```python
from build123d import *

# Parameters (mm, degrees)
F0_W      = 23.876
F0_H      = 22.352
F1_DEPTH  = 31.75
F2_R      = 0.796109
F3_DEPTH  = 25.4
F5_R      = 0.835635
F6_DEPTH  = 6.35
F7_R      = 0.804369
F4_W      = 23.876
F4_H      = 22.352
F4_R      = 0.796109
F8_DEPTH  = 6.35
F9_R      = 43.215518
F10_DEPTH = 127


with BuildPart() as f1:
    # F0 (on Top) → F1 (new body)
    with BuildSketch(Plane.XY):
        with Locations((11.938, -11.176)):
            Rectangle(F0_W, F0_H)
    extrude(amount=F1_DEPTH)

    # F2 (on face) → F3 (cut)
    with BuildSketch(Plane.XY.offset(31.75)):
        with Locations((22.537371, -1.488913)):
            Circle(F2_R)
    extrude(amount=-F3_DEPTH, mode=Mode.SUBTRACT)

    # F5 (on face) → F6 (cut)
    with BuildSketch(Plane.XY.offset(31.75)):
        with Locations((1.065723, -1.193718)):
            Circle(F5_R)
    extrude(amount=-F6_DEPTH, mode=Mode.SUBTRACT)

    # F7 (on face) + F4 (on face) → F8 (cut)
    with BuildSketch(Plane.XY.offset(31.75)):
        with Locations((1.000239, -21.275662)):
            Circle(F7_R)
    with BuildSketch(Plane.XY.offset(31.75)):
        with Locations((11.938, -11.176)):
            Rectangle(F4_W, F4_H)
        with Locations((22.537371, -1.488913)):
            Circle(F4_R, mode=Mode.SUBTRACT)
    extrude(amount=-F8_DEPTH, mode=Mode.SUBTRACT)

    # F9 (on Front) → F10 (join)
    with BuildSketch(Plane.XZ):
        with Locations((32.045215, 28.994571)):
            Circle(F9_R)
    extrude(amount=F10_DEPTH)


solid = f1.part
```
The listing builds one solid part. Answer for the finished solid, in the listing's coordinates (mm). Give positions to 0.01 mm unless a question says otherwise; leave off trailing zeros. Order: outer loops, then holes, each group sorted by start corner. A loop starts at its lowest first (then second) coordinate and runs counter-clockwise, first axis right, second up. Notation, with made-up numbers: (63, 54.5) -> (87, 54.5) arc R13 cw to (87, 65.5) -> close; hole circle Ø2 at (-2.5, -6.75). An arc over 180 degrees is marked (long way). Write each question's results on one line, items separated by ' | '.
Q1. Each of these flat-tipped pins is pushed along its axis until it touches: P1, Ø1.5, axis at x = 39.5, y = -105.5, coming from the -Z side; P2, Ø1.5, axis at x = 60, y = -90.5, coming from the +Z side; P3, Ø4, axis at x = 13, y = -60.5, coming from the -Z side. Where does it stop, or does it pass through?
Checked values:
P1: stops at z = -13.7 | P2: stops at z = 62.57 | P3: stops at z = -10.72
Q2. The part is cut by section C-C, the plane y = -30. Give the vertices of the cut face in (x, z), and give its area (3 significant figures).
Checked values:
outline: circle Ø86.43 at (32.05, 28.99) | area: 5,870 mm^2
Q3. Straight lines are drawn through the part: probe 1 along Z at (x, y) = (33, -75); probe 2 along X at (y, z) = (-54.5, 8.5); probe 3 along Z at (x, y) = (43, -39.5). For each, find the intervals that lie inside material, in ascending order. Write a range as from..to.
Checked values:
probe 1: z = -14.21..72.2 | probe 2: x = -6..70.09 | probe 3: z = -12.81..70.8
Q4. The part is cut by section B-B, the plane z = 43.5. Give the vertices of the cut face in (x, y), and give its area (3 significant figures).
Checked values:
outline: (-8.66, -127) -> (72.75, -127) -> (72.75, 0) -> (-8.66, 0) -> close | area: 10,300 mm^2
Q5. The part is cut by section A-A, the plane x = 69.5. Give the vertices of the cut face in (y, z), and give its area (3 significant figures).
Checked values:
outline: (-127, 7.44) -> (0, 7.44) -> (0, 50.55) -> (-127, 50.55) -> close | area: 5,480 mm^2
